```python
from build123d import *

# Parameters (mm, degrees)
F0_W        = 5
F0_H        = 2
F1_DEPTH    = 3
F2_R        = 2
F3_DEPTH    = 5
F4_W        = 218.5
F4_H        = 33.5
F5_DEPTH    = 2
F6_W        = 13.5
F6_H        = 5
F7_DEPTH    = 25
F8_T1_DEPTH = 5


# Not quite as in the source:
# - a fillet or chamfer that OpenCascade refuses, or shapes differently, is made with other operations: its cross-section is extruded or revolved along the edge and cut away or added
# - a feature names something its author has since deleted; it is built from what else it names


with BuildPart() as f1:
    # F0 (on Front) → F1 (new body)
    with BuildSketch(Plane.XZ):
        Polygon((111.25, 5), (111.25, 18.75), (-111.25, 18.75), (-111.25, 5), (-111.25, -5), (-111.25, -18.75), (111.25, -18.75), (111.25, -5), align=None)
        with Locations((0, -12.25)):
            Rectangle(F0_W, F0_H, mode=Mode.SUBTRACT)
        with BuildLine():
            Line((-47.6515307717, 12.5), (-9, 12.5))
            ThreePointArc((-9, 12.5), (-6.1715728753, 11.3284271247), (-5, 8.5))
            Line((-5, 8.5), (-5, -8.5))
            ThreePointArc((-5, -8.5), (-6.1715728753, -11.3284271247), (-9, -12.5))
            Line((-9, -12.5), (-47.6515307717, -12.5))
            ThreePointArc((-47.6515307717, -12.5), (-55, -14.5), (-62.3484692283, -12.5))
            Line((-62.3484692284, -12.5), (-101, -12.5))
            ThreePointArc((-101, -12.5), (-103.8284271247, -11.3284271247), (-105, -8.5))
            Line((-105, -8.5), (-105, 8.5))
            ThreePointArc((-105, 8.5), (-103.8284271247, 11.3284271247), (-101, 12.5))
            Line((-101, 12.5), (-62.3484692284, 12.5))
            ThreePointArc((-62.3484692283, 12.5), (-55, 14.5), (-47.6515307717, 12.5))
        make_face(mode=Mode.SUBTRACT)
        with BuildLine():
            Line((62.3484692283, 12.5), (101, 12.5))
            ThreePointArc((101, 12.5), (103.8284271247, 11.3284271247), (105, 8.5))
            Line((105, 8.5), (105, -8.5))
            ThreePointArc((105, -8.5), (103.8284271247, -11.3284271247), (101, -12.5))
            Line((101, -12.5), (62.3484692283, -12.5))
            ThreePointArc((62.3484692283, -12.5), (55, -14.5), (47.6515307717, -12.5))
            Line((47.6515307716, -12.5), (9, -12.5))
            ThreePointArc((9, -12.5), (6.1715728753, -11.3284271247), (5, -8.5))
            Line((5, -8.5), (5, 8.5))
            ThreePointArc((5, 8.5), (6.1715728753, 11.3284271247), (9, 12.5))
            Line((9, 12.5), (47.6515307716, 12.5))
            ThreePointArc((47.6515307717, 12.5), (55, 14.5), (62.3484692283, 12.5))
        make_face(mode=Mode.SUBTRACT)
        with Locations((0, 12.25)):
            Rectangle(F0_W, F0_H, mode=Mode.SUBTRACT)
        with BuildLine():
            ThreePointArc((111.25, -5), (116.25, 0), (111.25, 5))
            Line((111.25, 5), (111.25, -5))
        make_face()
        with BuildLine():
            Line((-111.25, -5), (-111.25, 5))
            ThreePointArc((-111.25, 5), (-116.25, 0), (-111.25, -5))
        make_face()
    extrude(amount=F1_DEPTH)

    # F2 (on face) → F3 (join)
    with BuildSketch(Plane.XZ.offset(3)):
        with BuildLine():
            ThreePointArc((111.25, -5), (116.25, 0), (111.25, 5))
            Line((111.25, 5), (111.25, 18.75))
            Line((111.25, 18.75), (-111.25, 18.75))
            Line((-111.25, 18.75), (-111.25, 5))
            ThreePointArc((-111.25, 5), (-116.25, 0), (-111.25, -5))
            Line((-111.25, -5), (-111.25, -18.75))
            Line((-111.25, -18.75), (111.25, -18.75))
            Line((111.25, -18.75), (111.25, -5))
        make_face()
        with Locations((-111.25, 0)):
            Circle(F2_R, mode=Mode.SUBTRACT)
        with BuildLine():
            Line((-107.25, 15.75), (107.25, 15.75))
            ThreePointArc((107.25, 15.75), (107.9571067812, 15.4571067812), (108.25, 14.75))
            Line((108.25, 14.75), (108.25, -14.75))
            ThreePointArc((108.25, -14.75), (107.9571067812, -15.4571067812), (107.25, -15.75))
            Line((107.25, -15.75), (-107.25, -15.75))
            ThreePointArc((-107.25, -15.75), (-107.9571067812, -15.4571067812), (-108.25, -14.75))
            Line((-108.25, -14.75), (-108.25, 14.75))
            ThreePointArc((-108.25, 14.75), (-107.9571067812, 15.4571067812), (-107.25, 15.75))
        make_face(mode=Mode.SUBTRACT)
        with Locations((111.25, 0)):
            Circle(F2_R, mode=Mode.SUBTRACT)
    extrude(amount=F3_DEPTH)

    # F4 (on face) → F5 (join)
    with BuildSketch(Plane.XZ.offset(8)):
        Rectangle(F4_W, F4_H)
        with BuildLine():
            ThreePointArc((-108.25, 14.75), (-107.9571067812, 15.4571067812), (-107.25, 15.75))
            Line((-107.25, 15.75), (107.25, 15.75))
            ThreePointArc((107.25, 15.75), (107.9571067812, 15.4571067812), (108.25, 14.75))
            Line((108.25, 14.75), (108.25, -14.75))
            ThreePointArc((108.25, -14.75), (107.9571067812, -15.4571067812), (107.25, -15.75))
            Line((107.25, -15.75), (-107.25, -15.75))
            ThreePointArc((-107.25, -15.75), (-107.9571067812, -15.4571067812), (-108.25, -14.75))
            Line((-108.25, -14.75), (-108.25, 14.75))
        make_face(mode=Mode.SUBTRACT)
    extrude(amount=F5_DEPTH)

    # F6 (on face) → F7 (cut)
    with BuildSketch(Plane(origin=(0, 0, -18.75), x_dir=(1, 0, 0), z_dir=(0, 0, -1))):
        with Locations((-55, 7.5)):
            Rectangle(F6_W, F6_H)
        with Locations((55, 7.5)):
            Rectangle(F6_W, F6_H)
    extrude(amount=-F7_DEPTH, mode=Mode.SUBTRACT)

    # F8: fillet of radius 3.5 on 2 edges, made by hand

    # F8_s2 → F8_t1 (cut)
    with BuildSketch(Plane.YZ.offset(-2.5)):
        with BuildLine():
            ThreePointArc((0, 7.7858983849), (-0.8542486889, 10.0771862323), (-3, 11.25))
            Line((-3, 11.25), (0, 11.25))
            Line((0, 11.25), (0, 7.7858983849))
        make_face()
        with BuildLine():
            ThreePointArc((0, -7.7858983849), (-0.8542486889, -10.0771862323), (-3, -11.25))
            Line((-3, -11.25), (0, -11.25))
            Line((0, -11.25), (0, -7.7858983849))
        make_face()
    extrude(amount=F8_T1_DEPTH, mode=Mode.SUBTRACT)


solid = f1.part
```
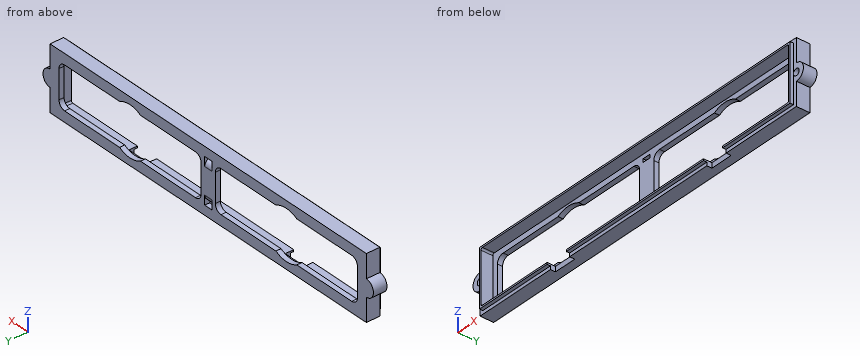
The listing builds one solid part. Answer for the finished solid, in the listing's coordinates (mm). Coordinates: 2 decimals unless noted, no trailing zeros. Loops run counter-clockwise (first coordinate to the right, second up) from the corner with the lowest first, then second, coordinate; pieces in that order, holes last. Notation, with made-up numbers: (-22, -39.5) - (33, -39.5) arc R32 cw to (33, -12.5) - close; hole circle Ø6 at (-15.5, 76.25). An arc over 180 degrees is marked (long way). Use a Markdown table: item, result. Add a question column.
1) The part is cut by section A-A, the plane x = -16.5. Give the vertices of the cut face in (y, z), and give its area (3 significant figures).
2) Find the intervals of material crossed by line 1 (X direction, y = -1.75, z = -7); line 2 (Z direction, x = -56, y = -3.5); line 3 (Z direction, x = 17.5, y = -2.25), in increasing order.
3) Given pin 1 (2.5 mm diameter, centred on x = 53.5, z = -17.5, fed in from -Y); pin 2 (1 mm diameter, centred on y = -2.5, z = -14.5, fed in from +X); pin 3 (2.5 mm diameter, centred on y = -5, z = 12, fed in from -X); pin 4 (12 mm diameter, centred on x = -41.5, z = 2.5, fed in from +Y), each flat-ended and moving along its own axis, determine where each tip first touches the part or whether it passes through.
Here are the results:
| question | item | result |
|---|---|---|
| 1 | outline | (-10, -16.75) - (-8, -16.75) - (-8, -18.75) - (0, -18.75) - (0, -12.5) - (-3, -12.5) - (-3, -15.75) - (-10, -15.75) - close; (-10, 15.75) - (-3, 15.75) - (-3, 12.5) - (0, 12.5) - (0, 18.75) - (-8, 18.75) - (-8, 16.75) - (-10, 16.75) - close |
| 1 | area | 71.5 mm^2 |
| 2 | line 1 | x = -111.25 to -105, -5 to 5, 105 to 111.25 |
| 2 | line 2 | z = -18.75 to -15.75, 15.75 to 18.75 |
| 2 | line 3 | z = -18.75 to -12.5, 12.5 to 18.75 |
| 3 | pin 1 | stops at y = -5 |
| 3 | pin 2 | stops at x = 111.25 |
| 3 | pin 3 | stops at x = -111.25 |
| 3 | pin 4 | passes through |
